```python
from build123d import *

# Parameters (mm, degrees)
F2_DEPTH = 0.7
F3_DEPTH = 0.35
F5_D     = 4.2
F6_DEPTH = 1.25
F7_DEPTH = 30


with BuildPart() as f1:
    # F0 (on Front) → F1 (revolve)
    with BuildSketch(Plane.XZ):
        Polygon((-16, 84), (-16, 68), (16, 68), (16, 84), (16.35, 84), (16.35, 88), (-16.35, 88), (-16.35, 84), align=None)
    revolve(axis=Axis((-7.2666932824, 0, 0), (1, 0, 0)))

    # F2 (cut): a face of the model
    f2_faces = [f1.faces().sort_by_distance(p)[0] for p in [
        (16.35, 0, -86.4890158698),
    ]]
    extrude(f2_faces, amount=-F2_DEPTH, mode=Mode.SUBTRACT)

    # F3 (add): a face of the model
    f3_faces = [f1.faces().sort_by_distance(p)[0] for p in [
        (15.65, 0, -86.4890158698),
    ]]
    extrude(f3_faces, amount=F3_DEPTH)

    # F5 (through all)
    with Locations(Plane.YZ.offset(16)):
        with Locations((-67.6927920079, 39.7484076433), (0, 78.5), (67.6927920079, 39.7484076433), (68.5497314523, -38.2515923567), (0, -78.5), (-68.5497314523, -38.2515923567)):
            Hole(F5_D / 2)

    # F6 (add): a face of the model
    f6_faces = [f1.faces().sort_by_distance(p)[0] for p in [
        (-16.35, 0, -85.5109841302),
    ]]
    extrude(f6_faces, amount=F6_DEPTH)

    # F7 (cut): a face of the model
    f7_faces = [f1.faces().sort_by_distance(p)[0] for p in [
        (16, 0, -85.5109841302),
    ]]
    extrude(f7_faces, amount=-F7_DEPTH, mode=Mode.SUBTRACT)


solid = f1.part
```
Build history of the part. All positions in model axes, mm. A direction names the side the tool comes from. Give positions to 0.01 mm unless a question says otherwise; leave off trailing zeros. Loops run counter-clockwise (first coordinate to the right, second up) from the corner with the lowest first, then second, coordinate; pieces in that order, holes last. Notation, with made-up numbers: (-32, 85.25) -> (18, 85.25) arc R14 cw to (18, 111.25) -> close; hole circle Ø1 at (-26.75, 58.25). An arc over 180 degrees is marked (long way). One line per question, with ' | ' between items. Start each with the question number.
1) Two-plate mould, pull along Y, no slides. Class faces 3 (the flat face through (-14, -20, 66)), 4 (the cylindrical face through (-15.014, 1.666, -79.778)), 5 (the cylindrical face through (-15.775, 85.907, -19.077)): released by +Y, released by -Y, zero draft, split by the parting line, or undercut.
2) Cut at A-A (y = 0). Give the cut face in (x, z), plus the area to 3 significant figures.
3) Cut at B-B (z = -78.5). Give the cut face in (x, y).
4) Pin check, flat tips, straight feed: pin 1 (6.5 mm diameter, centred on y = -67.69, z = 39.75, fed in from +X); pin 2 (1.5 mm diameter, centred on x = -16, z = -21, fed in from +Y); pin 3 (1.5 mm diameter, centred on x = -15.5, z = -42.5, fed in from +Y); pin 4 (1 mm diameter, centred on x = -17, z = -39.5, fed in from +Y). Stop position of each tip, or through.
5) Cut at C-C (y = 28). Give the cut face in (x, z).
6) Probe L1, parallel to Z at x = -15.55, y = 0; L2, parallel to Y at x = -14.2, z = -39; L3, parallel to Y at x = -17.4, z = -60. List the from-to ranges inside material, lowest first.
7) 3-axis set-ups, long thin cutter, end or side, ignore diameter. For faces 1 (the cylindrical face through (-15.014, 1.666, 77.222)), 2 (the flat face through (-16, 68, 6)): which of +Z, -Z, +X, -X, +Y, -Y reach the whole face in a straight line?
Return value:
1) face 3: zero draft | face 4: undercut | face 5: split by the parting line
2) outline: (-17.6, -88) -> (-14, -88) -> (-14, -80.6) -> (-16, -80.6) -> (-16, -84) -> (-17.6, -84) -> close; (-17.6, 84) -> (-16, 84) -> (-16, 80.6) -> (-14, 80.6) -> (-14, 88) -> (-17.6, 88) -> close; (-16, -76.4) -> (-14, -76.4) -> (-14, -68) -> (-16, -68) -> close; (-16, 68) -> (-14, 68) -> (-14, 76.4) -> (-16, 76.4) -> close | area: 76.0 mm^2
3) outline: (-17.6, -39.77) -> (-14, -39.77) -> (-14, -2.1) -> (-16, -2.1) -> (-16, -29.9) -> (-17.6, -29.9) -> close; (-17.6, 29.9) -> (-16, 29.9) -> (-16, 2.1) -> (-14, 2.1) -> (-14, 39.77) -> (-17.6, 39.77) -> close
4) pin 1: x = -14 | pin 2: y = 85.64 | pin 3: y = 77.47 | pin 4: y = 78.89
5) outline: (-17.6, -83.43) -> (-14, -83.43) -> (-14, -61.97) -> (-16, -61.97) -> (-16, -79.2) -> (-17.6, -79.2) -> close; (-17.6, 79.2) -> (-16, 79.2) -> (-16, 61.97) -> (-14, 61.97) -> (-14, 83.43) -> (-17.6, 83.43) -> close
6) L1: -88 to -80.6, -76.4 to -68, 68 to 76.4, 80.6 to 88 | L2: -78.89 to -70.51, -66.59 to -55.7, 55.7 to 66.59, 70.51 to 78.89 | L3: -64.37 to -58.79, 58.79 to 64.37
7) face 1: +X, -X | face 2: -X
